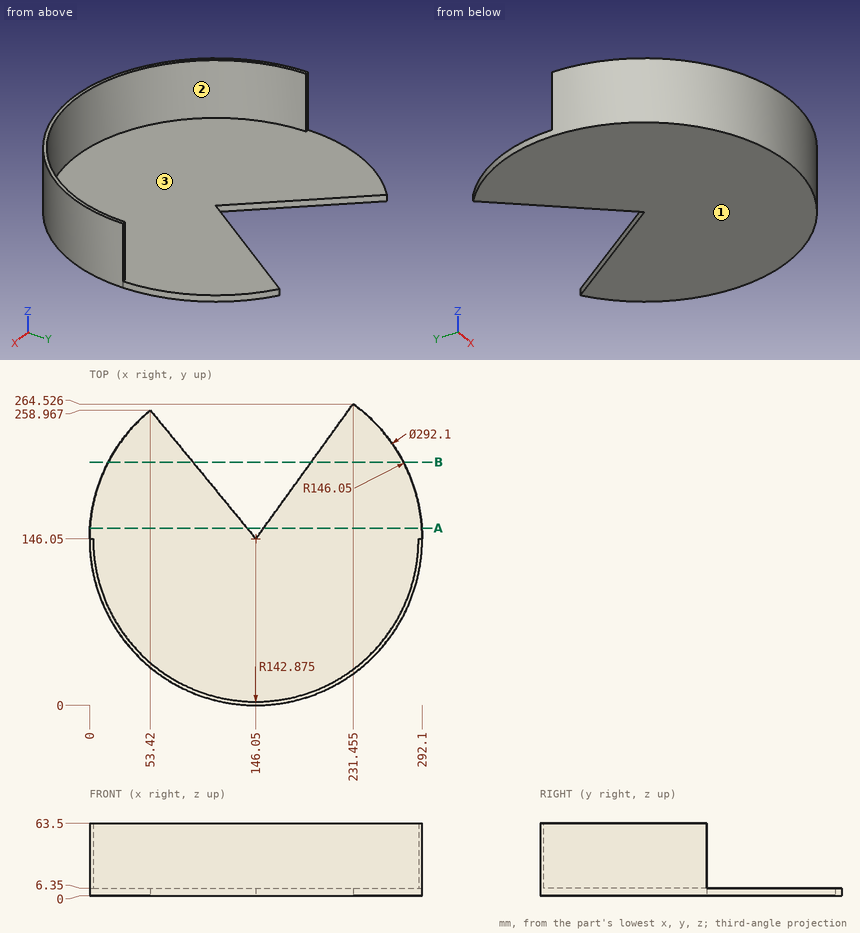
Drawing for the job (mm, zero at the part's lowest x, y, z). Round coordinates to 2 decimals unless told otherwise and drop trailing zeros. Loops run counter-clockwise (first coordinate to the right, second up) from the corner with the lowest first, then second, coordinate; pieces in that order, holes last. Notation, with made-up numbers: (66, -14.75) - (99, -14.75) arc R12 ccw to (99, -3.75) - close; hole circle Ø2 at (-34.5, 71). An arc over 180 degrees is marked (long way). Return JSON: item names as keys, results as strings. Group by question number.
Q1. Flat gauge pins, fed straight in: pin 1 Ø1.5 at (x, z) = (70, 11.5) entering from -Y; pin 2 Ø1.6 at (x, z) = (290, 28) entering from +Y; pin 3 Ø6 at (y, z) = (114, 47.5) entering from +X. Where does each tip first touch, or does it go through?
Q2. Drill centre lines: line 1 along Z through (x, y) = (222, 197); line 2 along X through (y, z) = (87.5, 22); line 3 along X through (y, z) = (24, 18.5) (1 decimal). Where is each one in solid material? Low to high. Write a range as [from, to].
Q3. Band-saw the part on B-B on y = 213.5. Give the cut face in (x, z).
Q4. Two-plate mould, pull along X, no slides. Class the marked faces 1, 2 and 3: +X half, -X half, draft (parallel to the pull), parting line (faces both ways), or undercut.
Q5. Band-saw the part on A-A on y = 155.5. Give the cut face in (x, z), plus the area to 3 significant figures.
Solutions:
{
 "1": {"pin 1": "stops at y = 20.91", "pin 2": "stops at y = 146.05", "pin 3": "stops at x = 289.18"},
 "2": {"line 1": "z = [0, 6.35]", "line 2": "x = [12.25, 15.72], [276.38, 279.85]", "line 3": "x = [65.8, 71.8], [220.3, 226.3]"},
 "3": {"outline": "(16.51, 0) - (90.72, 0) - (90.72, 6.35) - (16.51, 6.35) - close; (194.67, 0) - (275.59, 0) - (275.59, 6.35) - (194.67, 6.35) - close"},
 "4": {"face 1": "draft", "face 2": "undercut", "face 3": "undercut"},
 "5": {"outline": "(0.31, 0) - (138.3, 0) - (138.3, 6.35) - (0.31, 6.35) - close; (152.86, 0) - (291.79, 0) - (291.79, 6.35) - (152.86, 6.35) - close", "area": "1,760 mm^2"}
}
